Part model, mm, in its own coordinate system. A direction names the side the tool comes from. Round coordinates to 2 decimals unless told otherwise and drop trailing zeros. Order: outer loops, then holes, each group sorted by start corner. A loop starts at its lowest first (then second) coordinate and runs counter-clockwise, first axis right, second up. Notation, with made-up numbers: (-14.5, -3) - (14.5, -3) arc R26 ccw to (14.5, 16) - close; hole circle Ø1 at (9.25, 47.25). An arc over 180 degrees is marked (long way). Answer as a JSON object with one key per item and string values.
```python
from build123d import *

# Parameters (mm, degrees)
LASER_HOLES_R       = 124
LASER_HOLES_R_2     = 1.65
LASER_HOLES_R_3     = 12.15
BOSS_EXTRUDE4_DEPTH = 5


with BuildPart() as part:
    # Laser holes → Boss-Extrude4 (new body)
    with BuildSketch(Plane(origin=(0, 0, 0), x_dir=(1, 0, 0), z_dir=(0, 1, 0))):
        with Locations(Location((-49.5, 0, 0), (0, 0, 270))):
            Circle(LASER_HOLES_R)
        with Locations(Location((15.5, 15.5, 0), (0, 0, 270))):
            Circle(LASER_HOLES_R_2, mode=Mode.SUBTRACT)
        with Locations(Location((-15.5, 15.5, 0), (0, 0, 90))):
            Circle(LASER_HOLES_R_2, mode=Mode.SUBTRACT)
        with Locations(Location((-15.5, -15.5, 0), (0, 0, 270))):
            Circle(LASER_HOLES_R_2, mode=Mode.SUBTRACT)
        with Locations(Location((15.5, -15.5, 0), (0, 0, 90))):
            Circle(LASER_HOLES_R_2, mode=Mode.SUBTRACT)
        with Locations(Location((-31.82233047, 17.67766953, 0), (0, 0, 270))):
            Circle(LASER_HOLES_R_2, mode=Mode.SUBTRACT)
        with Locations(Location((-67.17766953, 17.67766953, 0), (0, 0, 270))):
            Circle(LASER_HOLES_R_2, mode=Mode.SUBTRACT)
        with Locations(Location((-67.17766953, -17.67766953, 0), (0, 0, 270))):
            Circle(LASER_HOLES_R_2, mode=Mode.SUBTRACT)
        with Locations(Location((-31.82233047, -17.67766953, 0), (0, 0, 270))):
            Circle(LASER_HOLES_R_2, mode=Mode.SUBTRACT)
        with Locations(Location((-49.5, 0, 0), (0, 0, 270))):
            Circle(LASER_HOLES_R_3, mode=Mode.SUBTRACT)
        with Locations(Location((-153.5, 11.2, 0), (0, 0, 270))):
            Circle(LASER_HOLES_R_2, mode=Mode.SUBTRACT)
        with Locations(Location((-153.5, -11.2, 0), (0, 0, 90))):
            Circle(LASER_HOLES_R_2, mode=Mode.SUBTRACT)
        with Locations(Location((-7.199484522, 95.666641994, 0), (0, 0, 90))):
            Circle(LASER_HOLES_R_2, mode=Mode.SUBTRACT)
        with Locations(Location((12.199484522, 84.466641994, 0), (0, 0, 270))):
            Circle(LASER_HOLES_R_2, mode=Mode.SUBTRACT)
        with Locations(Location((12.199484522, -84.466641994, 0), (0, 0, 90))):
            Circle(LASER_HOLES_R_2, mode=Mode.SUBTRACT)
        with Locations(Location((-7.199484522, -95.666641994, 0), (0, 0, 270))):
            Circle(LASER_HOLES_R_2, mode=Mode.SUBTRACT)
        with BuildLine():
            Line((14.5, -7), (14.5, 7))
            ThreePointArc((14.5, 7), (12.303300859, 12.303300859), (7, 14.5))
            Line((7, 14.5), (-7, 14.5))
            ThreePointArc((-7, 14.5), (-12.303300859, 12.303300859), (-14.5, 7))
            Line((-14.5, 7), (-14.5, -7))
            ThreePointArc((-14.5, -7), (-12.303300859, -12.303300859), (-7, -14.5))
            Line((-7, -14.5), (7, -14.5))
            ThreePointArc((7, -14.5), (12.303300859, -12.303300859), (14.5, -7))
        make_face(mode=Mode.SUBTRACT)
    extrude(amount=BOSS_EXTRUDE4_DEPTH)


solid = part.part
```
Item 1: Cut at C-C (x = 0). Write the cut outline in (y, z).
Taken from the geometry:
{"outline": "(0, -113.69) - (5, -113.69) - (5, -14.5) - (0, -14.5) - close; (0, 14.5) - (5, 14.5) - (5, 113.69) - (0, 113.69) - close"}
Item 2: Cut at A-A (x = -49.5). Write the cut outline in (y, z), plus the area to 3 significant figures.
Taken from the geometry:
{"outline": "(0, -124) - (5, -124) - (5, -12.15) - (0, -12.15) - close; (0, 12.15) - (5, 12.15) - (5, 124) - (0, 124) - close", "area": "1,120 mm2"}
Item 3: Cut at D-D (z = -35). Write the cut outline in (x, y), plus the area to 3 significant figures.
Taken from the geometry:
{"outline": "(-168.46, 0) - (69.46, 0) - (69.46, 5) - (-168.46, 5) - close", "area": "1,190 mm2"}
Item 4: Drop flat-ended pins along their axis: P1, Ø2, axis at x = -31.82, z = -17.68, coming from the -Y side; P2, Ø1.5, axis at x = -2.5, y = 3, coming from the +Z side. Give the stop position or say it passes through.
Taken from the geometry:
{"P1": "through", "P2": "z = 115.05"}
Item 5: Probe L1, parallel to Z at x = -153.5, y = 3.1; L2, parallel to X at y = 1.6, z = 16.5; L3, parallel to X at y = 1.4, z = -9. List the from-to ranges inside material, lowest first. Write a range as from..to.
Taken from the geometry:
{"L1": "-67.53..-12.85, -9.55..9.55, 12.85..67.53", "L2": "-172.4..-68.33, -66.02..-32.98, -30.67..-16.81, -14.19..14.19, 16.81..73.4", "L3": "-173.17..-57.66, -41.34..-14.23, 14.23..74.17"}
Item 6: Two-plate mould, pull along X, no slides. Class faces 1 (the flat face through (-75, 5, -2)), 2 (the cylindrical face through (-124.952, 2.465, -98.402)), 3 (the cylindrical face through (-61.36, 2.46, -2.63)): pulls with the +X half, pulls with the -X half, needs draft (parallel to the pull), parting line crosses it, or undercut.
Taken from the geometry:
{"face 1": "needs draft", "face 2": "parting line crosses it", "face 3": "undercut"}
Item 7: Cut at B-B (y = 1.5). State how many separate pieces and enclosed holes the cut face has, plus the area to 3 significant figures.
Taken from the geometry:
{"separate pieces": "1", "enclosed holes": "16", "area": "46,900 mm2"}
Item 8: Tool access for faces 4 (the flat face through (-75, 0, -2)), 5 (the cylindrical face through (-12.245, 2.465, -12.361)): list every direction of +Z, -Z, +X, -X, +Y, -Y with a clear straight run to the whole face (end or side of a thin tool).
Taken from the geometry:
{"face 4": "+Z, -Z, +X, -X, -Y", "face 5": "+Y, -Y"}
